Solid Edge part; units mm, degrees
sketch "Sketch1" plane through (0, 0, 0) normal (1, 0, 0) x (0, 1, 0)
  circle A0 centre (0, 0) radius 10
  circle A1 centre (0, 0) radius 25
extrude "Protrusion1" add sketch "Sketch1" along normal blind 8
sketch "Sketch2" plane through (0, 0, 0) normal (-1, 0, 0) x (0, -1, 0)
  circle A0 centre (0, 0) radius 13
extrude "ExtrudedCutout_1" cut sketch "Sketch2" against normal blind 4.5
sketch "Sketch3" plane through (8, 0, 0) normal (1, 0, 0) x (0, 1, 0)
  circle A0 centre (-22, 0) radius 1.6
extrude "Cutout1" cut sketch "Sketch3" against normal up to next
pattern_circular "Pattern1" count 6 over 360 about axis through (8, 0, 0) along (-1, 0, 0) of "Cutout1"
CAD build for the part. Positions are in the model's coordinates, mm. A direction names the side the tool comes from. Coordinates: 2 decimals unless noted, no trailing zeros. Write each loop counter-clockwise with the first axis right and the second up, starting at its lowest first coordinate (ties: lowest second). Pieces come first, ordered by that corner, then holes. Notation, with made-up numbers: (56.25, 32) - (86.25, 32) arc R24 cw to (86.25, 44) - close; hole circle Ø8 at (-39, 46.5). An arc over 180 degrees is marked (long way). Use a Markdown table: item, result. Add a question column.
Item 1: 3-axis set-ups, long thin cutter, end or side, ignore diameter. For faces 5 (the face through (2.218, 10.316, -7.91)), 6 (the face through (4.06, 9.82, -17.97)): which of +Z, -Z, +X, -X, +Y, -Y reach the whole face in a straight line?
Item 2: Band-saw the part on D-D, the plane z = -19.5. Give the cut face in (x, y), and give its area (3 significant figures).
Item 3: Band-saw the part on A-A, the plane y = 0. Give the cut face in (x, z).
Item 4: Band-saw the part on B-B, the plane z = 0. Give the cut face in (x, y).
Item 5: Drill centre lines: L1, parallel to Y at x = 1.25, z = -18; L2, parallel to Z at x = 3.25, y = 11; L3, parallel to Z at x = 7.25, y = -10.5. Where is each one in solid material? Low to high. Write a range as from..to.
Item 6: Mould opens along Z. For faces 1 (the face through (4.5, 8, -7)), 2 (the face through (4.056, 20.474, -0.481)), 3 (the face through (8, 11, 0)), 4 (the face through (3.944, 23.846, -7.509)) say: pulls with the +Z half, pulls with the -Z half, needs draft (parallel to the pull), parting line crosses it, or undercut.
Item 7: Flat gauge pins, fed straight in: pin 1 (2 mm diameter, centred on x = 2, z = -8.5, fed in from +Y); pin 2 (1 mm diameter, centred on x = 2.5, y = -13.5, fed in from -Z); pin 3 (13 mm diameter, centred on y = -3, z = -3.5, fed in from -X). Where does each tip first touch, or does it go through?
Item 8: Band-saw the part on C-C, the plane x = 5.5. Give the cut face in (y, z), and give its area (3 significant figures).
Numbers:
| question | item | result |
|---|---|---|
| 1 | face 5 | -X |
| 1 | face 6 | +X, -X |
| 2 | outline | (0, -15.64) - (8, -15.64) - (8, -12.54) - (0, -12.54) - close; (0, -9.46) - (8, -9.46) - (8, 9.46) - (0, 9.46) - close; (0, 12.54) - (8, 12.54) - (8, 15.64) - (0, 15.64) - close |
| 2 | area | 201 mm2 |
| 3 | outline | (0, -25) - (8, -25) - (8, -10) - (4.5, -10) - (4.5, -13) - (0, -13) - close; (0, 13) - (4.5, 13) - (4.5, 10) - (8, 10) - (8, 25) - (0, 25) - close |
| 4 | outline | (0, -25) - (8, -25) - (8, -23.6) - (0, -23.6) - close; (0, -20.4) - (8, -20.4) - (8, -10) - (4.5, -10) - (4.5, -13) - (0, -13) - close; (0, 13) - (4.5, 13) - (4.5, 10) - (8, 10) - (8, 20.4) - (0, 20.4) - close; (0, 23.6) - (8, 23.6) - (8, 25) - (0, 25) - close |
| 5 | L1 | -17.35..-12.21, -9.79..9.79, 12.21..17.35 |
| 5 | L2 | -22.45..-20.65, -17.45..-6.93, 6.93..17.45, 20.65..22.45 |
| 5 | L3 | -22.69..-20.57, -17.53..17.53, 20.57..22.69 |
| 6 | face 1 | undercut |
| 6 | face 2 | undercut |
| 6 | face 3 | needs draft |
| 6 | face 4 | parting line crosses it |
| 7 | pin 1 | y = 23.85 |
| 7 | pin 2 | z = -21.35 |
| 7 | pin 3 | x = 4.5 |
| 8 | outline | circle Ø50 at (0, 0); hole circle Ø3.2 at (-22, 0); hole circle Ø3.2 at (-11, -19.05); hole circle Ø3.2 at (-11, 19.05); hole circle Ø20 at (0, 0); hole circle Ø3.2 at (11, -19.05); hole circle Ø3.2 at (11, 19.05); hole circle Ø3.2 at (22, 0) |
| 8 | area | 1,600 mm2 |
